Source: CAD feature listing. Evaluate the final solid. Frame: model axes, mm. A direction names the side the tool comes from. Coordinates: 2 decimals unless noted, no trailing zeros.
Item 1: Reachability of faces 1 (the flat face through (31.5, -41, 13)), 2 (the flat face through (1.5, 0, 7)), 3 (the cylindrical face through (36.76, -9.76, -2.17)), 4 (the cylindrical face through (20.93, 13.97, 44.35)) from +Z, -Z, +X, -X, +Y, -Y: full face, straight path, thin tool, end or side. Return the list, or none.
Item 2: Mould query, pull axis X, two halves, no side actions, for faces 5 (the cylindrical face through (9.41, -39.05, -8.67)), 6 (the flat face through (0, -9, 9)), 7 (the flat face through (37.5, 1, 11)), 8 (the cylindrical face through (34.47, 13.97, 44.35)). Classes: released by +X, released by -X, zero draft, split by the parting line, or undercut.
Item 3: Contact query for flat-ended pins moving along their axis: P1, Ø16, axis at y = 2.5, z = 0.5, coming from the +X side; P2, Ø10, axis at x = 10, y = 16, coming from the +Z side; P3, Ø10, axis at x = 17.5, z = 5, coming from the -Y side; P4, Ø18, axis at y = 0, z = 0, coming from the -X side. Output: stop coordinate, or through.
Item 4: Ray query, line 1 (X direction, y = 36.5, z = 26.5); line 2 (Y direction, x = 28, z = 0); line 3 (X direction, y = -39, z = 13.5). Return the intervals inside material, ascending.
from build123d import *


with BuildPart() as f1:
    # F0 (on Front) → F1 (revolve)
    with BuildSketch(Plane.XZ):
        with BuildLine():
            Line((0, 42), (0, 10))
            Line((0, 10), (1.5, 10))
            Line((1.5, 10), (1.5, 6))
            Line((1.5, 6), (36, 6))
            Line((36, 6), (36, 10))
            Line((36, 10), (37.5, 10))
            Line((37.5, 10), (37.5, 46))
            ThreePointArc((37.5, 46), (37.3535533906, 46.3535533906), (37, 46.5))
            Line((37, 46.5), (32, 46.5))
            ThreePointArc((32, 46.5), (31.6464466094, 46.3535533906), (31.5, 46))
            Line((31.5, 46), (31.5, 42.5))
            Line((31.5, 42.5), (26.5, 42.5))
            Line((26.5, 42.5), (26.5, 46))
            ThreePointArc((26.5, 46), (26.3535533906, 46.3535533906), (26, 46.5))
            Line((26, 46.5), (16, 46.5))
            Line((16, 46.5), (16, 40))
            Line((16, 40), (3, 40))
            Line((3, 40), (3, 42.5))
            Line((3, 42.5), (0.5, 42.5))
            ThreePointArc((0.5, 42.5), (0.1464466094, 42.3535533906), (0, 42))
        make_face()
    revolve(axis=Axis((18.75, 0, 0), (-1, 0, 0)))


solid = f1.part
Answer list:
1. face 1: none
1. face 2: -X
1. face 3: +X
1. face 4: +X, -X
2. face 5: undercut
2. face 6: released by -X
2. face 7: released by +X
2. face 8: zero draft
3. P1: stops at x = 37.5
3. P2: stops at z = 38.46
3. P3: stops at y = -46.5
3. P4: stops at x = 1.5
4. line 1: x = 16 to 26.5, 31.5 to 37.5
4. line 2: y = -42.5 to -6, 6 to 42.5
4. line 3: x = 0 to 3, 16 to 37.5
